Build history of the part. All positions in model axes, mm. Face numbers are marked on the shaded views. A direction names the side the tool comes from. Coordinates: 2 decimals unless noted, no trailing zeros. Write each loop counter-clockwise with the first axis right and the second up, starting at its lowest first coordinate (ties: lowest second). Pieces come first, ordered by that corner, then holes. Notation, with made-up numbers: (-37, -31.5) -> (-1, -31.5) arc R24 cw to (-1, -13.5) -> close; hole circle Ø7 at (23.25, 37). An arc over 180 degrees is marked (long way). Write each question's results on one line, items separated by ' | '. Start each with the question number.
Q1. Saw through at A-A on z = 0. Count the separate pieces of the cut face and the enclosed holes in it, and give its area (3 significant figures).
Q2. Tool access for the marked faces 5, 6 and 7: list every direction of +Z, -Z, +X, -X, +Y, -Y with a clear straight run to the whole face (end or side of a thin tool).
Q3. Saw through at B-B on x = 1.5. Give the cut face in (y, z), and give its area (3 significant figures).
Q4. Drill centre lines: line 1 (Y direction, x = -15, z = 1.75); line 2 (X direction, y = 3.5, z = 5); line 3 (X direction, y = 3, z = 3). Where is each one in solid material? Low to high.
Q5. Two-plate mould, pull along Y, no slides. Class the marked faces 1, 2, 3 and 4: released by +Y, released by -Y, zero draft, split by the parting line, or undercut.
Q6. Drop flat-ended pins along their axis: pin 1 Ø3 at (y, z) = (-0.5, -4) entering from -X; pin 2 Ø0.8 at (y, z) = (-1.5, 3) entering from -X; pin 3 Ø1.9 at (x, y) = (15.5, 2.5) entering from -Z. Give the stop position or say it passes through.
from build123d import *

# Parameters (mm, degrees)
F0_W     = 38
F0_H     = 14.5
F1_DEPTH = 2
F2_W     = 25.5
F2_H     = 12.5
F3_DEPTH = 1
F4_W     = 8
F4_H     = 14.5
F5_DEPTH = 8.5
F6_R     = 2.5
F7_DEPTH = 25
F9_DEPTH = 5
F10_R    = 3.99999


# Not quite as in the source:
# - a fillet or chamfer is up to 0.001 mm smaller than in the source, because OpenCascade refuses the exact size


with BuildPart() as f1:
    # F0 (on Front) → F1 (new body)
    with BuildSketch(Plane.XZ):
        Rectangle(F0_W, F0_H)
    extrude(amount=F1_DEPTH)

    # F2 (on face) → F3 (cut)
    with BuildSketch(Plane.XZ.offset(2)):
        Rectangle(F2_W, F2_H)
    extrude(amount=-F3_DEPTH, mode=Mode.SUBTRACT)

    # F4 (on face) → F5 (join)
    with BuildSketch(Plane(origin=(0, 0, 0), x_dir=(-1, 0, 0), z_dir=(0, 1, 0))):
        with Locations((15, 0)):
            Rectangle(F4_W, F4_H)
        with Locations((-15, 0)):
            Rectangle(F4_W, F4_H)
    extrude(amount=F5_DEPTH)

    # F6 (on face) → F7 (cut)
    with BuildSketch(Plane.XY.offset(7.25)):
        with Locations((-15, 4)):
            Circle(F6_R)
        with Locations((15, 4)):
            Circle(F6_R)
    extrude(amount=-F7_DEPTH, mode=Mode.SUBTRACT)

    # F8 (on face) → F9 (cut)
    with BuildSketch(Plane(origin=(0, 0, -7.25), x_dir=(1, 0, 0), z_dir=(0, 0, -1))):
        Polygon((-15, -7.6661742094), (-11.825, -5.8330871047), (-11.825, -2.1669128953), (-15, -0.3338257906), (-18.175, -2.1669128953), (-18.175, -5.8330871047), align=None)
        Polygon((15, -7.6661742094), (18.175, -5.8330871047), (18.175, -2.1669128953), (15, -0.3338257906), (11.825, -2.1669128953), (11.825, -5.8330871047), align=None)
    extrude(amount=-F9_DEPTH, mode=Mode.SUBTRACT)

    # F10 (radius 4 in the source; OpenCascade refuses exactly that, so slightly less here)
    f10_edges = [f1.edges().sort_by_distance(p)[0] for p in [
        (-19, -2, 0),
        (-19, 8.5, 0),
        (11, 8.5, 0),
        (19, -2, 0),
        (-11, 8.5, 0),
        (19, 8.5, 0),
    ]]
    fillet(f10_edges, radius=F10_R)


solid = f1.part
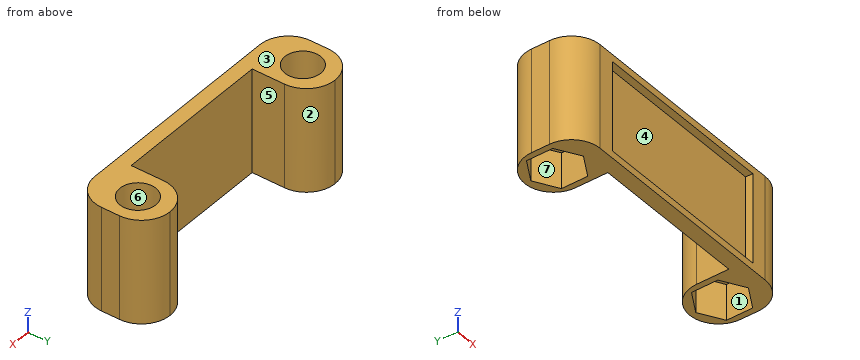
Returned:
1) separate pieces: 1 | enclosed holes: 2 | area: 127 mm2
2) face 5: +Z, -Z, +Y | face 6: +Z, -Z | face 7: -Z
3) outline: (-2, -7.25) -> (0, -7.25) -> (0, 7.25) -> (-2, 7.25) -> (-2, 6.25) -> (-1, 6.25) -> (-1, -6.25) -> (-2, -6.25) -> close | area: 16.5 mm2
4) line 1: y = -2 to 1.5, 6.5 to 8.5 | line 2: x = -19 to -17.45, -12.55 to -11, 11 to 12.55, 17.45 to 19 | line 3: x = -19 to -17.29, -12.71 to -11, 11 to 12.71, 17.29 to 19
5) face 1: undercut | face 2: released by +Y | face 3: zero draft | face 4: released by -Y
6) pin 1: stops at x = -18.87 | pin 2: stops at x = -17.53 | pin 3: stops at z = -2.25
